CAD build for the part. Positions are in the model's coordinates, mm. Round coordinates to 2 decimals unless told otherwise and drop trailing zeros. Order: outer loops, then holes, each group sorted by start corner. A loop starts at its lowest first (then second) coordinate and runs counter-clockwise, first axis right, second up.
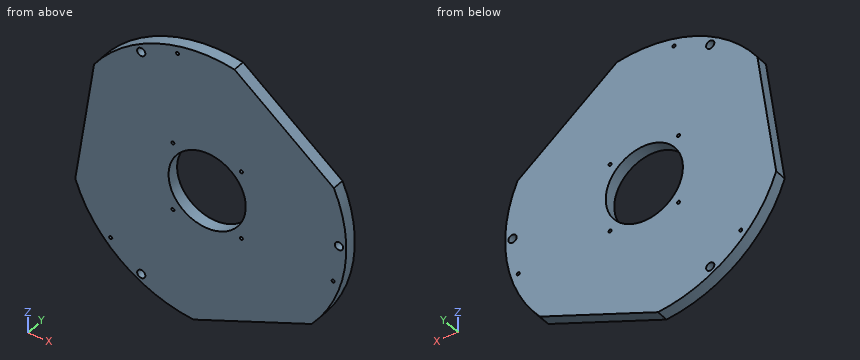
```python
from build123d import *

# Parameters (mm, degrees)
SKETCH1_W                    = 144.145
SKETCH1_H                    = 12.7
F_1_8_0_125_DIAMETER_HOLE1_D = 3.175
SKETCH4_OUTSIDE_W            = 371.87
SKETCH4_OUTSIDE_H            = 371.87
CUT_EXTRUDE1_DEPTH           = 205.247036821
SKETCH6_R                    = 40
CUT_EXTRUDE2_DEPTH           = 205.247036821
M10X1_5_TAPPED_HOLE1_D       = 8.5


with BuildPart() as part:
    # Sketch1 → Revolve1 (revolve)
    with BuildSketch(Plane.XY):
        with Locations((72.0725, -28.730222222)):
            Rectangle(SKETCH1_W, SKETCH1_H)
    revolve(axis=Axis((1e-09, -200000, 0), (0, 1, 0)))

    # 1/8 (0.125) Diameter Hole1 (through all)
    with Locations(Plane(origin=(0, -22.380222222, 0), x_dir=(1, 0, 0), z_dir=(0, 1, 0))):
        with Locations((136.525, 0), (-68.2625, -118.234118252), (-68.2625, 118.234118252), (-99.848064114, 93.109826108), (130.559506808, 39.916046987), (-30.711442694, -133.025873095), (-35.5, -35.5), (-35.5, 35.5), (35.5, 35.5), (35.5, -35.5)):
            Hole(F_1_8_0_125_DIAMETER_HOLE1_D / 2)

    # Sketch4 outside → Cut-Extrude1 (cut, through all)
    with BuildSketch(Plane(origin=(0, -22.380222222, 0), x_dir=(1, 0, 0), z_dir=(0, 1, 0))):
        Rectangle(SKETCH4_OUTSIDE_W, SKETCH4_OUTSIDE_H)
        Polygon((253.722129587, 37.919026331), (-94.022224704, -238.68932289), (-159.699904883, 200.770296559), align=None, mode=Mode.SUBTRACT)
    extrude(amount=-CUT_EXTRUDE1_DEPTH, mode=Mode.SUBTRACT)

    # Sketch6 → Cut-Extrude2 (cut, through all)
    with BuildSketch(Plane(origin=(0, -22.380222222, 0), x_dir=(1, 0, 0), z_dir=(0, 1, 0))):
        with Locations(Location((0, 0, 0), (0, 0, 180))):
            Circle(SKETCH6_R)
    extrude(amount=-CUT_EXTRUDE2_DEPTH, mode=Mode.SUBTRACT)

    # M10x1.5 Tapped Hole1 (through all)
    with Locations(Plane(origin=(0, -22.380222222, 0), x_dir=(1, 0, 0), z_dir=(0, 1, 0))):
        with Locations((-68.2625, 118.234118252), (136.525, 0), (-68.2625, -118.234118252)):
            Hole(M10X1_5_TAPPED_HOLE1_D / 2)


solid = part.part
```
1. Cut at A-A, the plane x = 0. Write the cut outline in (y, z) (3 decimals), and give its area (3 significant figures).
2. Cut at C-C, the plane y = -27.75. Give the number of separate pieces and of enclosed holes in the cut face, and give its area (3 significant figures).
3. Cut at B-B, the plane z = 16.5. Write the cut outline in (x, y).
4. Pin check, flat tips, straight feed: P1, Ø6, axis at y = -26, z = -12, coming from the -X side; P2, Ø3, axis at y = -27, z = 98, coming from the +X side; P3, Ø2, axis at y = -31.5, z = -22, coming from the -X side. Stop position of each tip, or through.
5. Cut at D-D, the plane x = 100.5. Write the cut outline in (y, z), and give its area (3 significant figures).
6. Drill centre lines: line 1 (X direction, y = -28.25, z = -30); line 2 (Z direction, x = 35.5, y = -27); line 3 (X direction, y = -27, z = 25). Where is each one in solid material? Low to high.
Outcome:
1. outline: (-35.08, -137.863) - (-22.38, -137.863) - (-22.38, -40) - (-35.08, -40) - close; (-35.08, 40) - (-22.38, 40) - (-22.38, 144.145) - (-35.08, 144.145) - close
1. area: 2,570 mm2
2. separate pieces: 1
2. enclosed holes: 11
2. area: 55,800 mm2
3. outline: (-127.23, -35.08) - (-36.44, -35.08) - (-36.44, -22.38) - (-127.23, -22.38) - close; (36.44, -35.08) - (143.2, -35.08) - (143.2, -22.38) - (36.44, -22.38) - close
4. P1: stops at x = -131.94
4. P2: stops at x = 84.73
4. P3: stops at x = -133.13
5. outline: (-35.08, -98.27) - (-22.38, -98.27) - (-22.38, 83.96) - (-35.08, 83.96) - close
5. area: 2,310 mm2
6. line 1: x = -134.18 to -26.46, 26.46 to 140.99
6. line 2: z = -123.88 to -37.09, -33.91 to -18.43, 18.43 to 33.91, 37.09 to 135.66
6. line 3: x = -125.96 to -31.22, 31.22 to 141.96
